from build123d import *

# Parameters (mm, degrees)
SCHIZZO1_R                   = 4.5
SCHIZZO1_R_2                 = 4
ESTRUSIONE_ESTRUSIONE1_DEPTH = 5
SCHIZZO2_R                   = 2
TAGLIO_ESTRUSIONE1_DEPTH     = 25


with BuildPart() as part:
    # Schizzo1 → Estrusione-Estrusione1 (new body)
    with BuildSketch(Plane.XY):
        with BuildLine():
            ThreePointArc((7.023974797, 138.427683332), (1.499753731, 147.278176914), (-7.525391936, 142.044153534))
            ThreePointArc((-7.525391936, 142.044153534), (-18.729107246, 69.99949188), (-12.22229981, -2.620188418))
            ThreePointArc((-12.22229981, -2.620188418), (3.068449146, -12.117533571), (11.996332959, 3.512548298))
            ThreePointArc((11.996332959, 3.512548298), (1.102237583, 70.660238267), (7.023974797, 138.427683332))
        make_face()
        Circle(SCHIZZO1_R, mode=Mode.SUBTRACT)
        with Locations((-0.309434746, 139.999658036)):
            Circle(SCHIZZO1_R_2, mode=Mode.SUBTRACT)
    extrude(amount=ESTRUSIONE_ESTRUSIONE1_DEPTH)

    # Schizzo2 → Taglio-Estrusione1 (cut)
    with BuildSketch(Plane.XY.offset(5)):
        with Locations((-6.142115432, 104.166670735)):
            Circle(SCHIZZO2_R)
        with Locations((-6.142115432, 32.213749463)):
            Circle(SCHIZZO2_R)
    extrude(amount=-TAGLIO_ESTRUSIONE1_DEPTH, mode=Mode.SUBTRACT)


solid = part.part
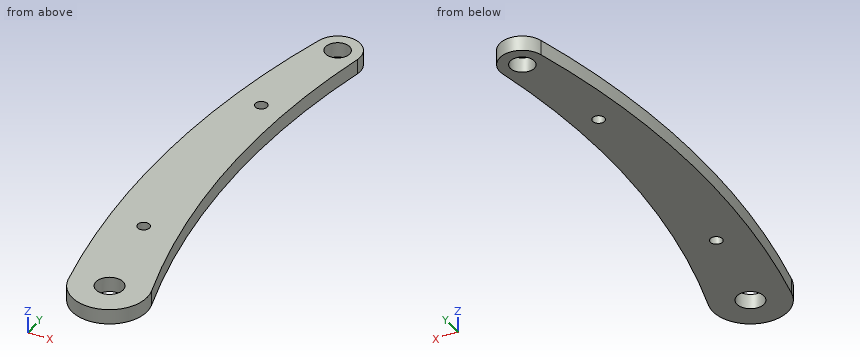
Verification items for the finished model (mm, model axes). Give positions to 0.01 mm unless a question says otherwise; leave off trailing zeros. Order: outer loops, then holes, each group sorted by start corner. A loop starts at its lowest first (then second) coordinate and runs counter-clockwise, first axis right, second up. Notation, with made-up numbers: M -18,10.25 L 25,10.25 A11 cw 25,30.25 Z; hole C 1.5,25 d8. An arc over 180 degrees is marked long. Answer as a JSON object with one key per item and string values. Group by question number.
1) Scan lines: line 1 along Y through (x, z) = (0, 3.1); line 2 along Y through (x, z) = (-1.5, 0.65); line 3 along X through (y, z) = (1.5, 3.9). Record each from-to range of solid material in increasing order. Write a range as [from, to].
2) Depth check by flat-ended pin: pin 1 Ø3 at (y, z) = (36, 3) entering from -X; pin 2 Ø3 at (y, z) = (105.5, 4) entering from -X; pin 3 Ø3 at (x, z) = (5, 3) entering from +Y. Enter the tip coordinate at first touch or a pass-through.
3) Cross-section at A-A (y = 0). Enter the section's corners in (x, z).
4) Cross-section at B-B (z = 3.75). Enter the section's corners in (x, y).
5) Cross-section at D-D (y = 70). Enter the section's corners in (x, z).
Result sheet:
{
 "1": {"line 1": "y = [-12.5, -4.5], [4.5, 136.01], [143.99, 147.49]", "line 2": "y = [-12.41, -4.24], [4.24, 136.18], [143.82, 147.4]", "line 3": "x = [-13.08, -4.24], [4.24, 12.41]"},
 "2": {"pin 1": "stops at x = -18.02", "pin 2": "stops at x = -15.68", "pin 3": "stops at y = 146.46"},
 "3": {"outline": "M -12.77,0 L -4.5,0 L -4.5,5 L -12.77,5 Z; M 4.5,0 L 12.5,0 L 12.5,5 L 4.5,5 Z"},
 "4": {"outline": "M -12.22,-2.62 A12.5 ccw long 12,3.51 A275 cw 7.02,138.43 A7.5 ccw -7.53,142.04 A300 ccw Z; hole C -6.14,32.21 d4; hole C -6.14,104.17 d4; hole C 0,0 d9; hole C -0.31,140 d8"},
 "5": {"outline": "M -18.73,0 L 1.13,0 L 1.13,5 L -18.73,5 Z"}
}
